Geometry: final body of the model. Coordinates: model frame, mm. A direction names the side the tool comes from. Give positions to 0.01 mm unless a question says otherwise; leave off trailing zeros. Order: outer loops, then holes, each group sorted by start corner. A loop starts at its lowest first (then second) coordinate and runs counter-clockwise, first axis right, second up. Notation, with made-up numbers: (86, 48) -> (98, 48) arc R13 ccw to (98, 61) -> close; hole circle Ø8 at (-16, 83). An arc over 180 degrees is marked (long way). Write item = value, one per line.
```python
from build123d import *

# Parameters (mm, degrees)
F1_DEPTH = 16
F2_R     = 1.5
F2_R_2   = 4.1
F3_DEPTH = 25.501
F5_DEPTH = 1


with BuildPart() as f1:
    # F0 (on Front) → F1 (new body)
    with BuildSketch(Plane.XZ):
        with BuildLine():
            ThreePointArc((77.1384719389, -108.9582770923), (94.3987552884, -94.3987552884), (108.9582770923, -77.1384719389))
            Line((108.9582770923, -77.1384719389), (106.8369567488, -75.0171515954))
            Line((106.8369567488, -75.0171515954), (75.0171515954, -106.8369567488))
            Line((75.0171515954, -106.8369567488), (77.1384719389, -108.9582770923))
        make_face()
    extrude(amount=F1_DEPTH)

    # F2 (on face) → F3 (cut, through all)
    with BuildSketch(Plane(origin=(90.9270541721, 0, -90.9270541721), x_dir=(0, -1, 0), z_dir=(-0.7071067812, 0, 0.7071067812))):
        with Locations((8, 11.25)):
            Circle(F2_R)
        with Locations((8, 0)):
            Circle(F2_R_2)
        with Locations((8, -11.25)):
            Circle(F2_R)
    extrude(amount=-F3_DEPTH, mode=Mode.SUBTRACT)

    # F4 (on face) → F5 (cut)
    with BuildSketch(Plane(origin=(90.9270541721, 0, -90.9270541721), x_dir=(0, -1, 0), z_dir=(-0.7071067812, 0, 0.7071067812))):
        Polygon((7.5967662116, 8.100280037), (10.5261206085, 9.3259293141), (10.929354397, 12.475649277), (8.4032337884, 14.399719963), (5.4738793915, 13.1740706859), (5.070645603, 10.024350723), align=None)
        Polygon((5.070645603, -12.475649277), (7.5967662116, -14.399719963), (10.5261206085, -13.1740706859), (10.929354397, -10.024350723), (8.4032337884, -8.100280037), (5.4738793915, -9.3259293141), align=None)
    extrude(amount=-F5_DEPTH, mode=Mode.SUBTRACT)

    # F7 (on mid) → F8 (revolve)
    with BuildSketch(Plane.XZ.offset(8)):
        with BuildLine():
            Line((88.522891116, -79.1890816044), (88.1693377254, -79.542634995))
            add(Edge.make_bspline(
                [(88.1693377254, -79.542634995), (86.9168482293, -80.7951244911), (88.7321185884, -82.9338429826), (90.290658069, -84.4923824633)],
                knots=[0, 0, 0, 0, 5.3851648071, 5.3851648071, 5.3851648071, 5.3851648071], degree=3))
            Line((90.290658069, -84.4923824633), (93.8261919749, -88.0279163692))
            Line((93.8261919749, -88.0279163692), (95.5939589279, -86.2601494162))
            Line((95.5939589279, -86.2601494162), (88.522891116, -79.1890816044))
        make_face()
    revolve(axis=Axis((87.3915202661, -8, -87.3915202661), (-0.7071067812, 0, 0.7071067812)))


solid = f1.part
```
1) Section query A-A (x = 104). Output: boundary loops of the cut face in (y, z), plus the area to 3 significant figures.
Check sheet entries:
outline = (-16, -83.7) -> (0, -83.7) -> (0, -77.85) -> (-16, -77.85) -> close
area = 93.6 mm²
2) Reachability of faces 1 (the face through (97.67, -7.89, -91.01)), 2 (the face through (85.12, -6.96, -97.43)), 3 (the face through (83.058, -10.725, -99.493)) from +Z, -Z, +X, -X, +Y, -Y: full face, straight path, thin tool, end or side. Return the list, or none.
Check sheet entries:
face_1 = -Z, +X, +Y, -Y
face_2 = -X
face_3 = none
3) Line query: line 1 (Z direction, x = 85, y = -6.25); line 2 (X direction, y = -11, z = -89.5); line 3 (X direction, y = -4.5, z = -82). Output: solid intervals per line, ascending. Write a range as from..to.
Check sheet entries:
line_1 = -102.94..-98.27, -97.73..-96.85, -94..-90.24
line_2 = 81.19..85.55, 93.45..99.06
line_3 = 86.74..89.91, 99.85..105.35
4) Section query B-B (z = -105). Output: boundary loops of the cut face in (x, y).
Check sheet entries:
outline = (76.85, -16) -> (82.45, -16) -> (82.45, 0) -> (76.85, 0) -> close
5) Mould query, pull axis X, two halves, no side actions, for faces 4 (the face through (99.79, -7.67, -85.95)), 5 (the face through (76.06, -7.89, -107.88)), 6 (the face through (92, 0, -92)). Classes: +X half, -X half, draft (parallel to the pull), parting line (faces both ways), or undercut.
Check sheet entries:
face_4 = undercut
face_5 = -X half
face_6 = draft
6) First-contact query: P1, Ø4, axis at y = -10.5, z = -86, coming from the -X side; P2, Ø5, axis at x = 90.5, z = -83.5, coming from the +Y side; P3, Ø3, axis at x = 100, y = -6.5, coming from the -Z side. Flat tips, straight axial feed; report the tip coordinate or a pass-through.
Check sheet entries:
P1 = 79.71
P2 = -1.87
P3 = -90.11
